Autodesk Inventor part; units mm, degrees
ref_plane "YZ Plane" through (0, 0, 0) normal (1, 0, 0) x (0, 1, 0)
ref_plane "XZ Plane" through (0, 0, 0) normal (0, 1, 0) x (-1, 0, 0)
ref_plane "XY Plane" through (0, 0, 0) normal (0, 0, 1) x (1, 0, 0)
sketch "Sketch1" plane through (0, 0, 0) normal (0, 0, 1) x (1, 0, 0)
  circle A0 centre (0, 12.7) radius 2.0828
  circle A1 centre (12.7, 0) radius 2.0828
  circle A2 centre (0, -12.7) radius 2.0828
  circle A3 centre (-12.7, 0) radius 2.0828
  arc A4 (5.5881, 19.3163) -> (4.8187, 19.5224) centre (0, 0) ccw
  circle A5 centre (0, 0) radius 20.1083
  line L0 (-1.5875, 1.3335) -> (-1.5875, -1.3335)
  line L1 (-1.3335, -1.5875) -> (1.3335, -1.5875)
  line L2 (1.5875, -1.3335) -> (1.5875, 1.3335)
  arc A6 (1.5875, 1.3335) -> (1.3335, 1.5875) centre (1.3335, 1.3335) ccw
  arc A7 (-1.3335, 1.5875) -> (-1.5875, 1.3335) centre (-1.3335, 1.3335) ccw
  arc A8 (-1.5875, -1.3335) -> (-1.3335, -1.5875) centre (-1.3335, -1.3335) ccw
  arc A9 (1.3335, -1.5875) -> (1.5875, -1.3335) centre (1.3335, -1.3335) ccw
  line L3 (-1.3335, 1.5875) -> (1.3335, 1.5875)
  point P0 (0, 0)
  point P1 (5.5881, 19.3163)
  point P2 (1.5875, 1.5875)
  point P3 (1.5875, 0)
  point P4 (0, -1.5875)
  point P5 (0, 1.5875)
  point P6 (4.8187, 19.5224)
  dimension "halfLength" = 1.5875
  dimension "d16" = 1.5875
  dimension "d17" = 1.5875
  dimension "d18" = 1.5875
  dimension "d20" = 0.254
  dimension "d21" = 2.667
  dimension "d22" = 2.667
  dimension "d23" = 40.2167
  dimension "d24" = 4.1656
  dimension "d25" = 4.1656
  dimension "d26" = 4.1656
  dimension "d27" = 4.1656
extrude "Extrusion3" add sketch "Sketch1" along normal blind 1.524
equation "\"d18\" = d17"
equation "\"d21\" = 2 * halfLength - 2 * d20"
equation "\"d22\" = d21"
equation "\"d25\" = d24"
equation "\"d26\" = d24"
equation "\"d27\" = d24"
properties part number "HS adapter retainer"
Build history of the part. All positions in model axes, mm. A direction names the side the tool comes from. Coordinates: 2 decimals unless noted, no trailing zeros. Write each loop counter-clockwise with the first axis right and the second up, starting at its lowest first coordinate (ties: lowest second). Pieces come first, ordered by that corner, then holes. Notation, with made-up numbers: (-40, -33) -> (8, -33) arc R27 ccw to (8, -16) -> close; hole circle Ø5 at (-19, -21.75). An arc over 180 degrees is marked (long way). Use CSV: the item, a comma, the result in double quotes. Start each with the question number.
Q1. 3-axis set-ups, long thin cutter, end or side, ignore diameter. For faces 1 (the flat face through (0, 1.588, 1)), 2 (the flat face through (0, -4, 1.524)): which of +Z, -Z, +X, -X, +Y, -Y reach the whole face in a straight line?
Q2. Pull direction Y, two halves, no side cores. Call faces 3 (the flat face through (0, -4, 0)), 4 (the cylindrical face through (14.687, -0.626, 0.751)): released by +Y, released by -Y, zero draft, split by the parting line, or undercut.
Q3. Cut at C-C, the plane y = 14. List the corners of the cut face in (x, z).
Q4. Cut at D-D, the plane y = 9. List the corners of the cut face in (x, z), then the cut area to 3 significant figures.
Q5. Cut at A-A, the plane x = 0. List the corners of the cut face in (y, z).
Q6. Flat gauge pins, fed straight in: pin 1 Ø3.5 at (x, y) = (0, 12.7) entering from -Z; pin 2 Ø0.5 at (x, z) = (-0.5, 0.5) entering from +Y. Where does each tip first touch, or does it go through?
Q7. Drill centre lines: probe 1 along Y at (x, z) = (0, 0.35); probe 2 along X at (y, z) = (1.5, 1.3); probe 3 along X at (y, z) = (-1, 1.2). Where is each one in solid material? Low to high.
Q8. Cut at B-B, the plane x = 12.7. List the corners of the cut face in (y, z).
Checked values:
1,face 1,"+Z, -Z"
1,face 2,"+Z, +X, -X, +Y, -Y"
2,face 3,"zero draft"
2,face 4,"undercut"
3,outline,"(-14.43, 0) -> (-1.63, 0) -> (-1.63, 1.52) -> (-14.43, 1.52) -> close; (1.63, 0) -> (14.43, 0) -> (14.43, 1.52) -> (1.63, 1.52) -> close"
4,outline,"(-17.98, 0) -> (17.98, 0) -> (17.98, 1.52) -> (-17.98, 1.52) -> close"
4,area,"54.8 mm²"
5,outline,"(-20.11, 0) -> (-14.78, 0) -> (-14.78, 1.52) -> (-20.11, 1.52) -> close; (-10.62, 0) -> (-1.59, 0) -> (-1.59, 1.52) -> (-10.62, 1.52) -> close; (1.59, 0) -> (10.62, 0) -> (10.62, 1.52) -> (1.59, 1.52) -> close; (14.78, 0) -> (20.11, 0) -> (20.11, 1.52) -> (14.78, 1.52) -> close"
6,pin 1,"passes through"
6,pin 2,"stops at y = 20.11"
7,probe 1,"y = -20.11 to -14.78, -10.62 to -1.59, 1.59 to 10.62, 14.78 to 20.11"
7,probe 2,"x = -20.05 to -14.15, -11.25 to -1.53, 1.53 to 11.25, 14.15 to 20.05"
7,probe 3,"x = -20.08 to -14.53, -10.87 to -1.59, 1.59 to 10.87, 14.53 to 20.08"
8,outline,"(-15.59, 0) -> (-2.08, 0) -> (-2.08, 1.52) -> (-15.59, 1.52) -> close; (2.08, 0) -> (15.59, 0) -> (15.59, 1.52) -> (2.08, 1.52) -> close"
